Read the model definition and answer for the solid it produces. Units are mm, in the model's axes. A direction names the side the tool comes from. Coordinates: 2 decimals unless noted, no trailing zeros. Loops run counter-clockwise (first coordinate to the right, second up) from the corner with the lowest first, then second, coordinate; pieces in that order, holes last. Notation, with made-up numbers: (26, -28.75) - (66, -28.75) arc R22 ccw to (66, -22.75) - close; hole circle Ø3 at (4.25, 37). An arc over 180 degrees is marked (long way). Use one line per item in the form item = value.
Autodesk Inventor part; units mm, degrees
ref_plane "YZ Plane" through (0, 0, 0) normal (1, 0, 0) x (0, 1, 0)
ref_plane "XZ Plane" through (0, 0, 0) normal (0, 1, 0) x (-1, 0, 0)
ref_plane "XY Plane" through (0, 0, 0) normal (0, 0, 1) x (1, 0, 0)
sketch "Sketch1" plane through (0, 0, 0) normal (0, 0, 1) x (1, 0, 0)
  line L0 (-35.56, 0) -> (35.56, 0)
  line L1 (0, -17.78) -> (0, 17.78)
  line L2 (-25.4, 12.7) -> (25.4, 12.7)
  line L3 (25.4, 12.7) -> (25.4, -12.7)
  line L4 (25.4, -12.7) -> (-25.4, -12.7)
  line L5 (-25.4, -12.7) -> (-25.4, 12.7)
  line L6 (22.225, 9.525) -> (-22.225, 9.525)
  line L7 (-22.225, 9.525) -> (-22.225, -9.525)
  line L8 (-22.225, -9.525) -> (22.225, -9.525)
  line L9 (22.225, -9.525) -> (22.225, 9.525)
  point P0 (0, 0)
  point P1 (-25.4, 0)
  point P2 (0, 12.7)
  dimension "d0" = 25.4
  dimension "d1" = 3.175
  dimension "d7" = 50.8
extrude "Extrusion1" add sketch "Sketch1" along normal mid plane 342.9 contours L5 L2 L1 L6 L7 L0 | L0 L7 L8 L1 L4 L5 | L1 L8 L9 L0 L3 L4 | L2 L3 L0 L9 L6 L1
properties part number "tubing_template_0.125" material "Aluminum-6061"
Item 1: Find the intervals of material crossed by L1, parallel to Y at x = 2, z = 67 (3 decimals); L2, parallel to X at y = 7.75, z = 152.5 (3 decimals), in increasing order.
Results below:
L1 = -12.7 to -9.525, 9.525 to 12.7
L2 = -25.4 to -22.225, 22.225 to 25.4
Item 2: Which of the six approach directions +Z, -Z, +X, -X, +Y, -Y give full straight-line access (tool end or side, diameter ignored) to faces 1 (the flat face through (-22.225, 0, -2)), 2 (the flat face through (25.4, 0, -2))?
Results below:
face_1 = +Z, -Z
face_2 = +Z, -Z, +X, +Y, -Y
Item 3: The part is cut by section A-A on z = 18. Give the vertices of the cut face in (x, y) (3 decimals).
Results below:
outline = (-25.4, -12.7) - (25.4, -12.7) - (25.4, 12.7) - (-25.4, 12.7) - close; hole (-22.225, -9.525) - (22.225, -9.525) - (22.225, 9.525) - (-22.225, 9.525) - close
Item 4: The part is cut by section B-B on y = 0. Give the vertices of the cut face in (x, z) (3 decimals).
Results below:
outline = (-25.4, -171.45) - (-22.225, -171.45) - (-22.225, 171.45) - (-25.4, 171.45) - close; (22.225, -171.45) - (25.4, -171.45) - (25.4, 171.45) - (22.225, 171.45) - close
Item 5: This flat-tipped pin is pushed along its axis until it touches: P1, Ø6, axis at x = -19, y = 0.5, coming from the -Z side. Where does it stop, or does it pass through?
Results below:
P1 = through
Item 6: For a pull along Y with two mould halves and no side action, classify faces 3 (the flat face through (-25.4, 0, -2)), 4 (the flat face through (0, 12.7, -2)), 5 (the flat face through (0, -12.7, -2)), 6 (the flat face through (0, 9.525, -2)) as +Y half, -Y half, draft (parallel to the pull), parting line (faces both ways), or undercut.
Results below:
face_3 = draft
face_4 = +Y half
face_5 = -Y half
face_6 = undercut
Item 7: The part is cut by section C-C on x = -18. Give the vertices of the cut face in (y, z) (3 decimals), plus the area to 3 significant figures.
Results below:
outline = (-12.7, -171.45) - (-9.525, -171.45) - (-9.525, 171.45) - (-12.7, 171.45) - close; (9.525, -171.45) - (12.7, -171.45) - (12.7, 171.45) - (9.525, 171.45) - close
area = 2,180 mm²
